Input: part model. Units: mm. Frame: model coordinates. Face numbers are marked on the shaded views. A direction names the side the tool comes from. Coordinates: 2 decimals unless noted, no trailing zeros. Loops run counter-clockwise (first coordinate to the right, second up) from the corner with the lowest first, then second, coordinate; pieces in that order, holes last.
Item 1: Reachability of the marked faces 1, 2 and 3 from +Z, -Z, +X, -X, +Y, -Y: full face, straight path, thin tool, end or side. Return the list, or none.
Item 2: Contact query for flat-ended pins moving along their axis: P1, Ø5, axis at x = 7, y = 14, coming from the -Z side; P2, Ø3, axis at x = 8, z = 5.5, coming from the +Y side; P3, Ø1.5, axis at x = 4, y = 26, coming from the -Z side. Output: stop coordinate, or through.
Item 3: Ray query, line 1 along Y through (x, z) = (7.75, 0); line 2 along Z through (x, y) = (3, 14); line 3 along Y through (x, z) = (7.75, -5). Return the intervals inside material, ascending.
Item 4: Section C-C on z = -10. Return loops of the section in (x, y).
Item 5: Section D-D on z = 26. Return loops of the section in (x, y), and give its area (3 significant figures).
Item 6: Section B-B on x = 6.25. Return loops of the section in (y, z).
Item 7: Section A-A on y = 23.75. Return loops of the section in (x, z).
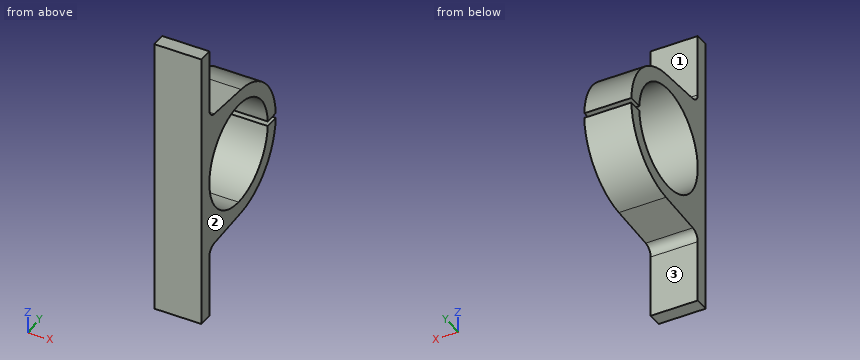
```python
from build123d import *

# Parameters (mm, degrees)
BOSS_EXTRUDE1_DEPTH     = 10
BOSS_EXTRUDE3_DEPTH     = 10
SKETCH5_W               = 10
SKETCH5_H               = 60
BOSS_EXTRUDE4_DEPTH     = 3
FILLET2_R               = 2
SKETCH2_R               = 11
ENL_V_MAT_EXTRU_1_DEPTH = 11
ESQUISSE3_W             = 1.042364678
ESQUISSE3_H             = 5.062914153
ENL_V_MAT_EXTRU_2_DEPTH = 11


with BuildPart() as part:
    # Sketch1 → Boss-Extrude1 (new body)
    with BuildSketch(Plane(origin=(0, 0, 0), x_dir=(0, 0, -1), z_dir=(1, 0, 0))):
        with BuildLine():
            Line((-15, 0), (15, 0))
            Line((15, 0), (9.520917343, 17.058125725))
            ThreePointArc((9.520917343, 17.058125725), (0, 24), (-9.520917343, 17.058125725))
            Line((-9.520917343, 17.058125725), (-15, 0))
        make_face()
    extrude(amount=BOSS_EXTRUDE1_DEPTH)

    # Sketch4 → Boss-Extrude3 (add)
    with BuildSketch(Plane(origin=(10, 0, 0), x_dir=(0, 0, -1), z_dir=(1, 0, 0))):
        with BuildLine():
            Line((9.520917343, 17.058125725), (15, 0))
            Line((15, 0), (13.966745843, 14.964370546))
            ThreePointArc((13.966745843, 14.964370546), (0, 28), (-13.966745843, 14.964370546))
            Line((-13.966745843, 14.964370546), (-15, 0))
            Line((-15, 0), (-9.520917343, 17.058125725))
            ThreePointArc((-9.520917343, 17.058125725), (0, 24), (9.520917343, 17.058125725))
        make_face()
    extrude(amount=-BOSS_EXTRUDE3_DEPTH)

    # Sketch5 → Boss-Extrude4 (add)
    with BuildSketch(Plane.XZ):
        with Locations((5, 0)):
            Rectangle(SKETCH5_W, SKETCH5_H)
    extrude(amount=-BOSS_EXTRUDE4_DEPTH)

    # Fillet2
    fillet2_edges = [part.edges().sort_by_distance(p)[0] for p in [
        (5, 3, -14.792857143),
        (5, 3, 14.792857143),
    ]]
    fillet(fillet2_edges, radius=FILLET2_R)

    # Sketch2 → Enlèv. mat.-Extru.1 (cut, through all)
    with BuildSketch(Plane(origin=(10, 0, 0), x_dir=(0, 0, -1), z_dir=(1, 0, 0))):
        with Locations((0, 14)):
            Circle(SKETCH2_R)
    extrude(amount=-ENL_V_MAT_EXTRU_1_DEPTH, mode=Mode.SUBTRACT)

    # Esquisse3 → Enlèv. mat.-Extru.2 (cut, through all)
    with BuildSketch(Plane(origin=(10, 0, 0), x_dir=(0, 0, -1), z_dir=(1, 0, 0))):
        with Locations((0, 26.657285384)):
            Rectangle(ESQUISSE3_W, ESQUISSE3_H)
    extrude(amount=-ENL_V_MAT_EXTRU_2_DEPTH, mode=Mode.SUBTRACT)


solid = part.part
```
Results found:
1. face 1: +Z, +X, -X, +Y
1. face 2: +Z, -Z, +X, +Y, -Y
1. face 3: -Z, +X, -X, +Y
2. P1: stops at z = -14.21
2. P2: stops at y = 27.42
2. P3: stops at z = -8.33
3. line 1: y = 0 to 3
3. line 2: z = -14.03 to -11, 11 to 14.03
3. line 3: y = 0 to 4.2, 23.8 to 27.08
4. outline: (0, 0) - (10, 0) - (10, 9.42) - (0, 9.42) - close; (0, 18.58) - (10, 18.58) - (10, 23.8) - (0, 23.8) - close
5. outline: (0, 0) - (10, 0) - (10, 3) - (0, 3) - close
5. area: 30.0 mm2
6. outline: (0, -30) - (3, -30) - (3, -16.66) arc R2 cw to (4.86, -14.66) - (14.96, -13.97) arc R14 ccw to (27.99, -0.52) - (24.99, -0.52) arc R11 cw (long way) to (24.99, 0.52) - (27.99, 0.52) arc R14 ccw to (14.96, 13.97) - (4.86, 14.66) arc R2 cw to (3, 16.66) - (3, 30) - (0, 30) - close
7. outline: (0, -10.05) - (10, -10.05) - (10, -5.09) - (0, -5.09) - close; (0, 5.09) - (10, 5.09) - (10, 10.05) - (0, 10.05) - close
